Drawing for the job (mm, zero at the part's lowest x, y, z). A direction names the side the tool comes from. Coordinates: 2 decimals unless noted, no trailing zeros. Write each loop counter-clockwise with the first axis right and the second up, starting at its lowest first coordinate (ties: lowest second). Pieces come first, ordered by that corner, then holes. Notation, with made-up numbers: M 77.5,76 L 117.5,76 A36 ccw 117.5,110 Z; hole C 4.5,4.25 d1. An arc over 180 degrees is marked long. Use a Markdown table: item, result. Add a question column.
Q1. Tool access for the marked faces 1, 2, 3, 4 and 5: list every direction of +Z, -Z, +X, -X, +Y, -Y with a clear straight run to the whole face (end or side of a thin tool).
Q2. Slice it at C-C on z = 10.05. Write the cut outline in (x, y).
Q3. Slice it at A-A on z = 15.6. Count the separate pieces of the cut face and the enclosed holes in it, then the cut area to 3 significant figures.
Q4. Wall check: L1, parallel to Y at x = 43.5, z = 14.5; L2, parallel to X at y = 11, z = 11; L3, parallel to Y at x = 51, z = 13.5. Give the ranges that are in metal, low to high. Write a range as from..to.
Q5. Slice it at B-B on x = 36.95. Write the cut outline in (y, z).
Q6. Pin check, flat tips, straight feed: pin 1 Ø5.5 at (x, z) = (49, 7.5) entering from +Y; pin 2 Ø10 at (y, z) = (23.5, 13) entering from -X; pin 3 Ø2 at (x, z) = (3.5, 12.5) entering from +Y. Stop position of each tip, or through.
Q7. Slice it at D-D on y = 39. Write the cut outline in (x, z).
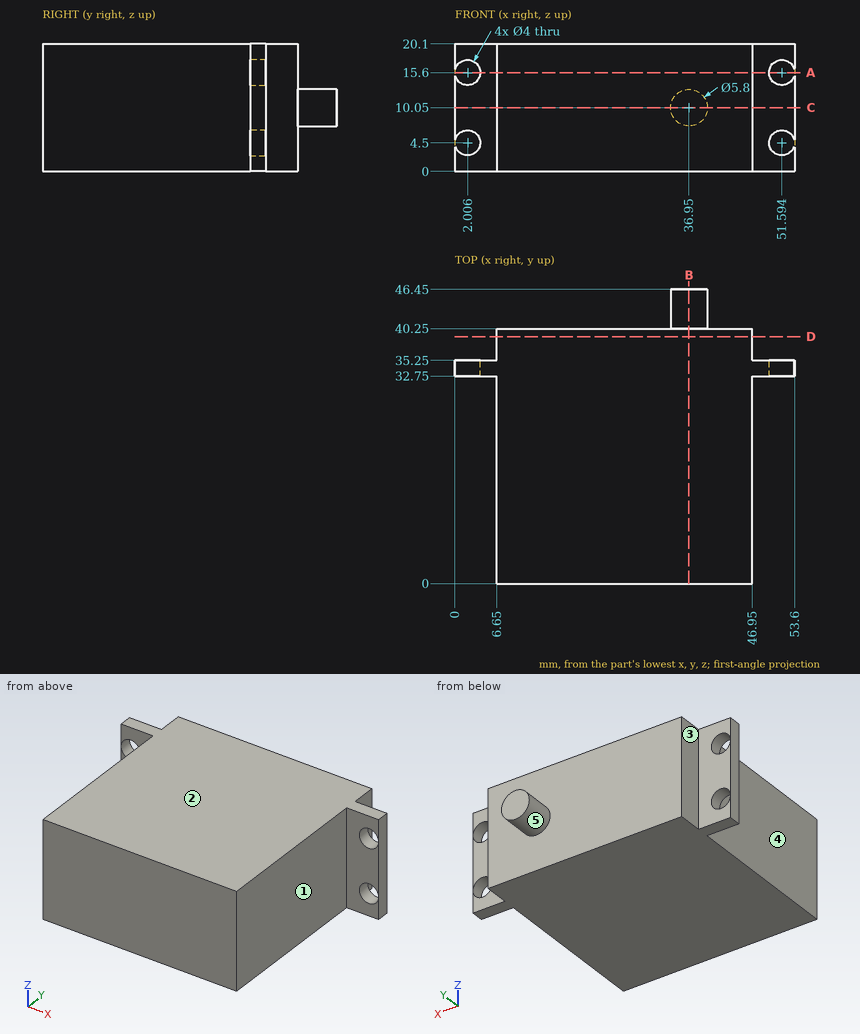
Recorded:
| question | item | result |
|---|---|---|
| 1 | face 1 | +Z, -Z, +X, -Y |
| 1 | face 2 | +Z, +X, -X, +Y, -Y |
| 1 | face 3 | +Z, -Z, -X, +Y |
| 1 | face 4 | +Z, -Z, -X, -Y |
| 1 | face 5 | +Y |
| 2 | outline | M 0,32.75 L 6.65,32.75 L 6.65,0 L 46.95,0 L 46.95,32.75 L 53.6,32.75 L 53.6,35.25 L 46.95,35.25 L 46.95,40.25 L 39.85,40.25 L 39.85,46.45 L 34.05,46.45 L 34.05,40.25 L 6.65,40.25 L 6.65,35.25 L 0,35.25 Z |
| 3 | separate pieces | 3 |
| 3 | enclosed holes | 0 |
| 3 | area | 1,640 mm² |
| 4 | L1 | 0..40.25 |
| 4 | L2 | 6.65..46.95 |
| 4 | L3 | 32.75..35.25 |
| 5 | outline | M 0,0 L 40.25,0 L 40.25,7.15 L 46.45,7.15 L 46.45,12.95 L 40.25,12.95 L 40.25,20.1 L 0,20.1 Z |
| 6 | pin 1 | y = 40.25 |
| 6 | pin 2 | x = 6.65 |
| 6 | pin 3 | y = 35.25 |
| 7 | outline | M 6.65,0 L 46.95,0 L 46.95,20.1 L 6.65,20.1 Z |
